```python
from build123d import *

# Parameters (mm, degrees)
SKETCH1_W                       = 20
SKETCH1_H                       = 60
BOSS_EXTRUDE1_DEPTH             = 10
SKETCH3_W                       = 20
SKETCH3_H                       = 3
BOSS_EXTRUDE2_DEPTH             = 20
BOSS_EXTRUDE2_DRAFT             = -3
BOSS_EXTRUDE2_PROFILE_2_DEPTH   = 20
BOSS_EXTRUDE2_PROFILE_2_DRAFT   = -3
FILLET1_R                       = 3
SKETCH7_W                       = 20
SKETCH7_H                       = 15
BOSS_EXTRUDE3_DEPTH             = 52
BOSS_EXTRUDE3_DIRECTION_2_REACH = 74.352
BOSS_EXTRUDE4_REACH             = 74.712
SKETCH11_W                      = 20
SKETCH11_H                      = 15
BOSS_EXTRUDE4_DIRECTION_2_DEPTH = 52
CUT_EXTRUDE2_START              = -20
CUT_EXTRUDE2_DEPTH              = 127.898033865


with BuildPart() as part:
    # Sketch1 → Boss-Extrude1 (new body)
    with BuildSketch(Plane.XY):
        with Locations((10, 30)):
            Rectangle(SKETCH1_W, SKETCH1_H)
    extrude(amount=BOSS_EXTRUDE1_DEPTH)


with BuildPart() as boss_extrude2_tool:
    # Sketch3 → Boss-Extrude2 (with draft: the straight prism first)
    with BuildSketch(Plane(origin=(0, 0, 0), x_dir=(-1, 0, 0), z_dir=(0, 0, -1))):
        with Locations((-10, 38.3)):
            Rectangle(SKETCH3_W, SKETCH3_H)
    extrude(amount=BOSS_EXTRUDE2_DEPTH)
    # Boss-Extrude2: the draft: its side faces are tilted about the plane it starts from
    boss_extrude2_sides = [boss_extrude2_tool.faces().sort_by_distance(p)[0] for p in [
        (20, 38.3, -10),
        (10, 36.8, -10),
        (0, 38.3, -10),
        (10, 39.8, -10),
    ]]
    draft(boss_extrude2_sides, Plane(origin=(0, 0, 0), x_dir=(-1, 0, 0), z_dir=(0, 0, -1)), BOSS_EXTRUDE2_DRAFT)


with BuildPart() as part_1:
    add(part.part)

    # Boss-Extrude2: add boss_extrude2_tool
    add(boss_extrude2_tool.part)


with BuildPart() as boss_extrude2_profile_2_tool:
    # Sketch3 → Boss-Extrude2 profile 2 (with draft: the straight prism first)
    with BuildSketch(Plane(origin=(0, 0, 0), x_dir=(-1, 0, 0), z_dir=(0, 0, -1))):
        with Locations((-10, 21.7)):
            Rectangle(SKETCH3_W, SKETCH3_H)
    extrude(amount=BOSS_EXTRUDE2_PROFILE_2_DEPTH)
    # Boss-Extrude2 profile 2: the draft: its side faces are tilted about the plane it starts from
    boss_extrude2_profile_2_sides = [boss_extrude2_profile_2_tool.faces().sort_by_distance(p)[0] for p in [
        (20, 21.7, -10),
        (10, 20.2, -10),
        (0, 21.7, -10),
        (10, 23.2, -10),
    ]]
    draft(boss_extrude2_profile_2_sides, Plane(origin=(0, 0, 0), x_dir=(-1, 0, 0), z_dir=(0, 0, -1)), BOSS_EXTRUDE2_PROFILE_2_DRAFT)


with BuildPart() as part_2:
    add(part_1.part)

    # Boss-Extrude2 profile 2: add boss_extrude2_profile_2_tool
    add(boss_extrude2_profile_2_tool.part)

    # Fillet1
    fillet1_edges = [part_2.edges().sort_by_distance(p)[0] for p in [
        (10, 36.8, 0),
        (10, 39.8, 0),
        (10, 20.2, 0),
        (10, 23.2, 0),
    ]]
    fillet(fillet1_edges, radius=FILLET1_R)

    # Sketch7 → Boss-Extrude3 (add)
    with BuildSketch(Plane(origin=(0, 10.232604755, 28.113850506), x_dir=(-1, 0, 0), z_dir=(0, 0.34202014332566943, 0.9396926207859081))):
        with Locations((-10, -8.113337756)):
            Rectangle(SKETCH7_W, SKETCH7_H)
    extrude(amount=BOSS_EXTRUDE3_DEPTH)

    # Boss-Extrude3 direction 2: up to this face of the body (flat: up to its plane)
    boss_extrude3_direction_2_end = Plane(part_2.part.faces().sort_by_distance((10, 30, 10))[0])
    # Sketch7 → Boss-Extrude3 direction 2 (add, up to the picked face)
    with BuildSketch(Plane(origin=(0, 10.232604755, 28.113850506), x_dir=(-1, 0, 0), z_dir=(0, 0.34202014332566943, 0.9396926207859081)), mode=Mode.PRIVATE) as boss_extrude3_direction_2_sk1:
        with Locations((-10, -8.113337756)):
            Rectangle(SKETCH7_W, SKETCH7_H)
    boss_extrude3_direction_2_tool1 = split(extrude(boss_extrude3_direction_2_sk1.sketch, amount=-BOSS_EXTRUDE3_DIRECTION_2_REACH, mode=Mode.PRIVATE), bisect_by=boss_extrude3_direction_2_end, keep=Keep.BOTH, mode=Mode.PRIVATE)
    add(boss_extrude3_direction_2_tool1.solids().sort_by(Axis((10, 17.856648, 25.338926), (0, -0.34202014332566943, -0.9396926207859081)))[0])

    # Boss-Extrude4: up to this plane
    boss_extrude4_end = Plane(origin=(0, 0, 10), z_dir=(0, 0, -1))
    # Sketch11 → Boss-Extrude4 (add, up to the surface)
    with BuildSketch(Plane(origin=(0, 10.232604755, 28.113850506), x_dir=(-1, 0, 0), z_dir=(0, 0.34202014332566943, 0.9396926207859081)), mode=Mode.PRIVATE) as boss_extrude4_sk1:
        with Locations((-10, -38.613337756)):
            Rectangle(SKETCH11_W, SKETCH11_H)
    boss_extrude4_tool1 = split(extrude(boss_extrude4_sk1.sketch, amount=-BOSS_EXTRUDE4_REACH, mode=Mode.PRIVATE), bisect_by=boss_extrude4_end, keep=Keep.BOTH, mode=Mode.PRIVATE)
    add(boss_extrude4_tool1.solids().sort_by_distance((10, 46.517273, 14.907311))[0])

    # Sketch11 → Boss-Extrude4 direction 2 (add)
    with BuildSketch(Plane(origin=(0, 10.232604755, 28.113850506), x_dir=(-1, 0, 0), z_dir=(0, 0.34202014332566943, 0.9396926207859081))):
        with Locations((-10, -38.613337756)):
            Rectangle(SKETCH11_W, SKETCH11_H)
    extrude(amount=BOSS_EXTRUDE4_DIRECTION_2_DEPTH)

    # Sketch9 → Cut-Extrude2 (cut)
    with BuildSketch(Plane.ZY.offset(CUT_EXTRUDE2_START)):
        Polygon((275.181377297, 111.452308492), (73.347891487, 37.990927379), (68.649428383, 36.280826662), (67.794378024, 38.630058214), (63.09591492, 36.919957498), (66.516116354, 27.52303129), (71.214579458, 29.233132007), (70.359529099, 31.582363559), (75.057992203, 33.292464275), (276.891478013, 106.753845388), (680.558449633, 253.676607614), (678.848348917, 258.375070718), align=None)
    cut_extrude2 = extrude(amount=CUT_EXTRUDE2_DEPTH, mode=Mode.SUBTRACT)

    # Mirror1: Cut-Extrude2 across plane
    add(cut_extrude2.mirror(Plane(origin=(0, 21.954356086, -7.990732128), x_dir=(0, 0.3420201433256692, 0.9396926207859082), z_dir=(0, -0.9396926207859083, 0.3420201433256692))), mode=Mode.SUBTRACT)


solid = part_2.part
```
CAD build for the part. Positions are in the model's coordinates, mm. A direction names the side the tool comes from. Give positions to 0.01 mm unless a question says otherwise; leave off trailing zeros. Write each loop counter-clockwise with the first axis right and the second up, starting at its lowest first coordinate (ties: lowest second). Pieces come first, ordered by that corner, then holes. Notation, with made-up numbers: (66, 16.5) -> (91, 16.5) arc R31 ccw to (91, 52.5) -> close; hole circle Ø10 at (51.25, -19.75). An arc over 180 degrees is marked (long way). Write each question's results on one line, items separated by ' | '.
1. Drop flat-ended pins along their axis: P1, Ø12, axis at x = 16, y = 64, coming from the -Z side; P2, Ø3.5, axis at x = 9.5, y = 2.5, coming from the +Z side; P3, Ø5, axis at x = 2.5, z = 49, coming from the +Y side. Give the stop position or say it passes through.
Geometry check:
P1: z = 0 | P2: z = 10 | P3: y = 67.82
2. Two-plate mould, pull along Y, no slides. Class faces 1 (the flat face through (10, 0, 5)), 2 (the flat face through (10, 38, -20)), 3 (the flat face through (10.14, 59.571, 65.493)), 4 (the flat face through (10.14, 28.366, 68.832)): pulls with the +Y half, pulls with the -Y half, needs draft (parallel to the pull), parting line crosses it, or undercut.
Geometry check:
face 1: pulls with the -Y half | face 2: needs draft | face 3: pulls with the +Y half | face 4: undercut
3. Cut at C-C, the plane y = 51. Write the cut outline in (x, z), then the cut area to 3 significant figures.
Geometry check:
outline: (0, 0) -> (20, 0) -> (20, 49.15) -> (0, 49.15) -> close | area: 983 mm²
4. Which spindle directions (+Z, -Z, +X, -X, +Y, -Y) get a long thin tool onto all of the face, cutting with end or side? Do faces 5 (the cylindrical face through (9.86, 19.19, -0.91)), 6 (the flat face through (10, 29, 10)), 7 (the flat face through (10.14, 61.9, 35.24)), 8 (the flat face through (10.14, 37.148, 71.032)). Say none if no direction does.
Geometry check:
face 5: +X, -X, -Y | face 6: +X, -X | face 7: +X, -X, +Y | face 8: +Z, +X, -X
5. Cut at B-B, the plane z = -14. Write the cut outline in (x, y).
Geometry check:
outline: (-0.73, 19.47) -> (20.73, 19.47) -> (20.73, 23.93) -> (-0.73, 23.93) -> close; (-0.73, 36.07) -> (20.73, 36.07) -> (20.73, 40.53) -> (-0.73, 40.53) -> close
6. Wall check: probe 1 along Y at (x, z) = (8, 56.5); probe 2 along Y at (x, z) = (19.5, 2); probe 3 along Y at (x, z) = (0.75, 69). Give the ranges that are in metal, low to high. Write a range as [from, to].
Geometry check:
probe 1: [21.22, 37.18], [53.67, 56.33], [66.98, 69.64] | probe 2: [0, 60] | probe 3: [25.77, 28.43], [36.41, 41.73]
7. Cut at D-D, the plane y = 63. Write the cut outline in (x, z), then the cut area to 3 significant figures.
Geometry check:
outline: (0, 38.26) -> (20, 38.26) -> (20, 53.6) -> (0, 53.6) -> close | area: 307 mm²
8. Cut at A-A, the plane z = 47.5. Write the cut outline in (x, y).
Geometry check:
outline: (0, 17.94) -> (20, 17.94) -> (20, 33.9) -> (0, 33.9) -> close; (0, 50.4) -> (20, 50.4) -> (20, 66.36) -> (0, 66.36) -> close
